Geometry check sheet. Reference: the model listing, model coordinates, mm. Face numbers are marked on the shaded views. A direction names the side the tool comes from. Round coordinates to 2 decimals unless told otherwise and drop trailing zeros. Order: outer loops, then holes, each group sorted by start corner. A loop starts at its lowest first (then second) coordinate and runs counter-clockwise, first axis right, second up. Notation, with made-up numbers: (-25.75, -29) - (-2.75, -29) arc R9 ccw to (-2.75, -23) - close; hole circle Ø7 at (-8, 76.5). An arc over 180 degrees is marked (long way). Write each question's results on one line, items separated by ' | '.
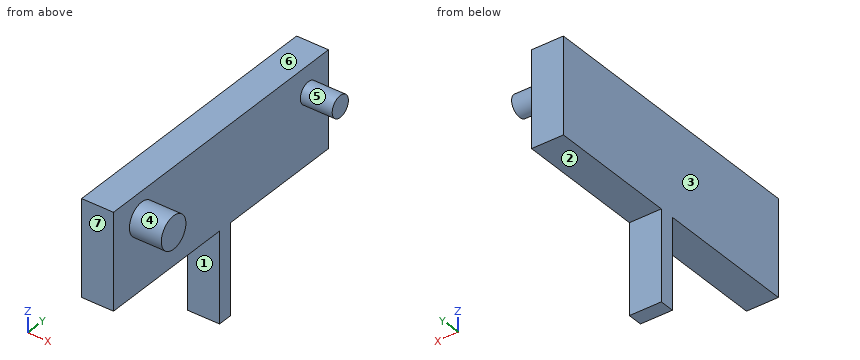
```python
from build123d import *

# Parameters (mm, degrees)
SKETCH1_R             = 2.55
BOSS_EXTRUDE1_DEPTH   = 10
SKETCH1_R_2           = 1.68
BOSS_EXTRUDE1_2_DEPTH = 10
SKETCH2_W             = 2.303802682
SKETCH2_H             = 14.158597278
SKETCH2_H_2           = 10.841402722
BOSS_EXTRUDE2_DEPTH   = 5


with BuildPart() as part:
    # Sketch1 → Boss-Extrude1 (new body)
    with BuildSketch(Plane.YZ):
        with Locations(Location((-75.554303292, 44.238232385, 0), (0, 0, 270))):
            Circle(SKETCH1_R)
    extrude(amount=BOSS_EXTRUDE1_DEPTH)



with BuildPart() as body_2:
    # Sketch1 → Boss-Extrude1 2 (new body)
    with BuildSketch(Plane.YZ):
        with Locations(Location((-40.954303292, 44.238232385, 0), (0, 0, 270))):
            Circle(SKETCH1_R_2)
    extrude(amount=BOSS_EXTRUDE1_2_DEPTH)


with BuildPart() as part_1:
    add(part.part)

    add(body_2.part)  # Boss-Extrude2 merges body 2
    # Sketch2 → Boss-Extrude2 (add)
    with BuildSketch(Plane.YZ):
        with Locations((-58.254303292, 26.317531024)):
            Rectangle(SKETCH2_W, SKETCH2_H)
        with Locations((-58.254303292, 38.817531024)):
            Rectangle(SKETCH2_W, SKETCH2_H_2)
        Polygon((-36.783173072, 48.461100861), (-81.407523603, 48.461100861), (-81.407523603, 33.396829663), (-59.406204633, 33.396829663), (-59.406204633, 44.238232385), (-57.102401951, 44.238232385), (-57.102401951, 33.396829663), (-36.783173072, 33.396829663), align=None)
    extrude(amount=BOSS_EXTRUDE2_DEPTH)


solid = part_1.part
```
(1) Material ranges on line 1 (Y direction, x = 3, z = 27.5); line 2 (X direction, y = -43, z = 44); line 3 (Z direction, x = 3.25, y = -65.5), recorded low to high.
Answers follow:
line 1: -59.41 to -57.1 | line 2: 0 to 5 | line 3: 33.4 to 48.46
(2) Section check C-C (y = -41.5). Record the cut outline in (x, z), then the cut area to 3 significant figures.
Answers follow:
outline: (0, 33.4) - (5, 33.4) - (5, 42.65) - (10, 42.65) - (10, 45.83) - (5, 45.83) - (5, 48.46) - (0, 48.46) - close | area: 91.2 mm²
(3) Section check A-A (x = 2). Record the cut outline in (y, z).
Answers follow:
outline: (-81.41, 33.4) - (-59.41, 33.4) - (-59.41, 19.24) - (-57.1, 19.24) - (-57.1, 33.4) - (-36.78, 33.4) - (-36.78, 48.46) - (-81.41, 48.46) - close
(4) Section check B-B (z = 43.5). Record the cut outline in (x, y).
Answers follow:
outline: (0, -81.41) - (5, -81.41) - (5, -78) - (10, -78) - (10, -73.11) - (5, -73.11) - (5, -42.46) - (10, -42.46) - (10, -39.45) - (5, -39.45) - (5, -36.78) - (0, -36.78) - close
(5) Depth check by flat-ended pin: pin 1 Ø4 at (x, z) = (3, 26.5) entering from +Y; pin 2 Ø6 at (y, z) = (-70, 39) entering from +X; pin 3 Ø5.5 at (x, y) = (3, -72.5) entering from -Z. Enter the tip coordinate at first touch or a pass-through.
Answers follow:
pin 1: y = -57.1 | pin 2: x = 5 | pin 3: z = 33.4
(6) Section check D-D (x = 6). Record the cut outline in (y, z).
Answers follow:
outline: circle Ø5.1 at (-75.55, 44.24); circle Ø3.36 at (-40.95, 44.24)
(7) Access from +Z, -Z, +X, -X, +Y, -Y to the whole of each face (thin tool, end or side, straight path). Record for the marked faces 1, 2 and 3.
Answers follow:
face 1: -Z, +X, -X, -Y | face 2: -Z, +X, -X, +Y | face 3: +Z, -Z, -X, +Y, -Y
(8) Draft check along Y on the marked faces 4, 5, 6 and 7. Enter one of: released by +Y, released by -Y, zero draft, split by the parting line, or undercut.
Answers follow:
face 4: undercut | face 5: undercut | face 6: zero draft | face 7: released by -Y
